Geometry check sheet. Reference: the model listing, model coordinates, mm. A direction names the side the tool comes from. Round coordinates to 2 decimals unless told otherwise and drop trailing zeros. Loops run counter-clockwise (first coordinate to the right, second up) from the corner with the lowest first, then second, coordinate; pieces in that order, holes last.
```python
from build123d import *

# Parameters (mm, degrees)
BOSS_EXTRUDE1_START            = -9
BOSS_EXTRUDE1_DEPTH            = 9
BOSS_EXTRUDE1_2_DEPTH          = 0.4
BOSS_EXTRUDE1_START_2          = -11.95
BOSS_EXTRUDE1_3_DEPTH          = 2.5
SKETCH2_W                      = 9
SKETCH2_H                      = 11
BOSS_EXTRUDE2_DEPTH            = 2.45
SKETCH3_W                      = 0.9
SKETCH3_H                      = 8.5
CUT_EXTRUDE1_DEPTH             = 20.892712233
SKETCH4_W                      = 0.52
SKETCH4_H                      = 6
CUT_EXTRUDE2_DEPTH             = 19.771520983
BOSS_EXTRUDE3_DEPTH            = 0.36
SKETCH6_W                      = 5.62
SKETCH6_H                      = 3
BOSS_EXTRUDE4_DEPTH            = 0.36
SKETCH7_W                      = 3
SKETCH7_H                      = 2.5
BOSS_EXTRUDE5_DEPTH            = 0.52
SKETCH8_W                      = 1.5
SKETCH8_H                      = 1.7
CUT_EXTRUDE3_DEPTH             = 20.7068516
SKETCH9_W                      = 6
SKETCH9_H                      = 1.5
BOSS_EXTRUDE6_DEPTH            = 1.5
SKETCH10_W                     = 10
SKETCH10_H                     = 4.5
CUT_EXTRUDE4_DEPTH             = 20.7068516
BOSS_EXTRUDE7_DEPTH            = 10
BOSS_EXTRUDE8_DEPTH            = 0.25
F_6_5_6_5_DIAMETER_HOLE1_D     = 6.5
F_6_5_6_5_DIAMETER_HOLE1_DEPTH = 7
SKETCH15_W                     = 6
SKETCH15_H                     = 1
SKETCH16_W                     = 0.75
SKETCH16_H                     = 7.825
F_1_5_1_5_DIAMETER_HOLE2_D     = 1.5
F_1_5_1_5_DIAMETER_HOLE3_D     = 1.5
F_1_5_1_5_DIAMETER_HOLE3_DEPTH = 13.88
CHAMFER1_SIZE                  = 0.2


with BuildPart() as part:
    # Boss-Extrude1: read off the stored shape, not the designer's step
    # Boss-Extrude1 outline → Boss-Extrude1 (new body)
    with BuildSketch(Plane(origin=(0, 0, -4.5), x_dir=(-1, 0, 0), z_dir=(0, 0, -1)).offset(BOSS_EXTRUDE1_START)):
        Polygon((11.95, -6.5), (11.95, 4.5), (0, 4.5), (0, -6.5), (9.45, -6.5), align=None)
    extrude(amount=BOSS_EXTRUDE1_DEPTH)

    # Boss-Extrude1 2 outline → Boss-Extrude1 2 (add)
    with BuildSketch(Plane(origin=(0, 0, -4.5), x_dir=(-1, 0, 0), z_dir=(0, 0, -1))):
        with BuildLine():
            Line((11.95, -8.75), (11.95, -6.5))
            Line((11.95, -6.5), (9.45, -6.5))
            Line((9.45, -6.5), (9.45, -8.75))
            ThreePointArc((9.45, -8.75), (10.7, -10), (11.95, -8.75))
        make_face()
    extrude(amount=BOSS_EXTRUDE1_2_DEPTH)

    # Boss-Extrude1 3 outline → Boss-Extrude1 3 (add)
    with BuildSketch(Plane.YZ.offset(BOSS_EXTRUDE1_START_2)):
        with BuildLine():
            Line((-6.5, -4.9), (-3.989897949, -4.9))
            ThreePointArc((-3.989897949, -4.9), (-3.673670183, -4.787298335), (-3.5, -4.5))
            Line((-3.5, -4.5), (-6.5, -4.5))
            Line((-6.5, -4.5), (-6.5, -4.9))
        make_face()
    extrude(amount=BOSS_EXTRUDE1_3_DEPTH)

    # Sketch2 → Boss-Extrude2 (add)
    with BuildSketch(Plane.ZY.offset(11.95)):
        with Locations((0, -1)):
            Rectangle(SKETCH2_W, SKETCH2_H)
    extrude(amount=BOSS_EXTRUDE2_DEPTH)

    # Sketch3 → Cut-Extrude1 (cut, through all)
    with BuildSketch(Plane.XY.offset(4.5)):
        with Locations((-13.95, 0.25)):
            Rectangle(SKETCH3_W, SKETCH3_H)
    extrude(amount=-CUT_EXTRUDE1_DEPTH, mode=Mode.SUBTRACT)

    # Sketch4 → Cut-Extrude2 (cut, through all)
    with BuildSketch(Plane.XZ.offset(6.5)):
        with Locations((-14.14, -1.5)):
            Rectangle(SKETCH4_W, SKETCH4_H)
    extrude(amount=-CUT_EXTRUDE2_DEPTH, mode=Mode.SUBTRACT)

    # Sketch5 → Boss-Extrude3 (add)
    with BuildSketch(Plane(origin=(-13.88, 0, 0), x_dir=(0, -1, 0), z_dir=(-1, 0, 0))):
        with BuildLine():
            Line((6.5, -1.5), (8.5, -1.5))
            ThreePointArc((8.5, -1.5), (10, 0), (8.5, 1.5))
            Line((8.5, 1.5), (6.5, 1.5))
            Line((6.5, 1.5), (6.5, -1.5))
        make_face()
    extrude(amount=-BOSS_EXTRUDE3_DEPTH)

    # Sketch6 → Boss-Extrude4 (add)
    with BuildSketch(Plane(origin=(-13.88, 0, 0), x_dir=(0, -1, 0), z_dir=(-1, 0, 0))):
        with Locations((1.19, 0)):
            Rectangle(SKETCH6_W, SKETCH6_H)
    extrude(amount=-BOSS_EXTRUDE4_DEPTH)

    # Sketch7 → Boss-Extrude5 (add)
    with BuildSketch(Plane.ZY.offset(13.88)):
        with Locations((-3, -5.25)):
            Rectangle(SKETCH7_W, SKETCH7_H)
    extrude(amount=BOSS_EXTRUDE5_DEPTH)

    # Sketch8 → Cut-Extrude3 (cut, through all)
    with BuildSketch(Plane(origin=(0, 0, -4.5), x_dir=(-1, 0, 0), z_dir=(0, 0, -1))):
        with Locations((1.75, 3.65)):
            Rectangle(SKETCH8_W, SKETCH8_H)
    extrude(amount=-CUT_EXTRUDE3_DEPTH, mode=Mode.SUBTRACT)

    # Sketch9 → Boss-Extrude6 (add)
    with BuildSketch(Plane(origin=(-2.5, 0, 0), x_dir=(0, 0, -1), z_dir=(1, 0, 0))):
        with Locations((0, 3.55)):
            Rectangle(SKETCH9_W, SKETCH9_H)
    extrude(amount=BOSS_EXTRUDE6_DEPTH)

    # Sketch10 → Cut-Extrude4 (cut, through all)
    with BuildSketch(Plane(origin=(0, 0, -4.5), x_dir=(-1, 0, 0), z_dir=(0, 0, -1))):
        with Locations((8.5, 2.25)):
            Rectangle(SKETCH10_W, SKETCH10_H)
    extrude(amount=-CUT_EXTRUDE4_DEPTH, mode=Mode.SUBTRACT)

    # Sketch11 → Boss-Extrude7 (add)
    with BuildSketch(Plane.ZY.offset(3.5)):
        with BuildLine():
            Line((4.1, 0), (-4.1, 0))
            ThreePointArc((-4.1, 0), (0, 4.1), (4.1, 0))
        make_face()
    extrude(amount=BOSS_EXTRUDE7_DEPTH)

    # Sketch12 → Boss-Extrude8 (add)
    with BuildSketch(Plane(origin=(-7.825, 0, 0), x_dir=(0, -1, 0), z_dir=(-1, 0, 0))):
        with BuildLine():
            Line((8.75, 1.25), (6.5, 1.25))
            Line((6.5, 1.25), (6.5, -1.25))
            Line((6.5, -1.25), (8.75, -1.25))
            ThreePointArc((8.75, -1.25), (10, 0), (8.75, 1.25))
        make_face()
    extrude(amount=-BOSS_EXTRUDE8_DEPTH)

    # Ø6.5 (6.5) Diameter Hole1
    with Locations(Plane(origin=(0, 0, 0), x_dir=(0, 0, -1), z_dir=(1, 0, 0))):
        with Locations((0, 0)):
            Hole(F_6_5_6_5_DIAMETER_HOLE1_D / 2, depth=F_6_5_6_5_DIAMETER_HOLE1_DEPTH)

    # Sketch15 → Revolve1 (revolve)
    with BuildSketch(Plane.XY, mode=Mode.PRIVATE) as revolve1_sk:
        with Locations((-4, 0.5)):
            Rectangle(SKETCH15_W, SKETCH15_H)
    revolve(revolve1_sk.sketch.rotate(Axis((-7, 0, 0), (1, 0, 0)), 270), axis=Axis((-7, 0, 0), (1, 0, 0)))

    # Sketch16 → Ø1.5 (1.5) Diameter Hole1 (revolve, cut)
    with BuildSketch(Plane(origin=(-7.825, -8.75, 0), x_dir=(0, 0, 1), z_dir=(0, 1, 0))):
        with Locations((0.375, 3.9125)):
            Rectangle(SKETCH16_W, SKETCH16_H)
    revolve(axis=Axis((-14.175, -8.75, 0), (1, 0, 0)), mode=Mode.SUBTRACT)

    # Ø1.5 (1.5) Diameter Hole2 (through all)
    with Locations(Plane.XY.offset(-4.5)):
        with Locations((-10.7, -8.75)):
            Hole(F_1_5_1_5_DIAMETER_HOLE2_D / 2)

    # Ø1.5 (1.5) Diameter Hole3
    with Locations(Plane.ZY.offset(13.88)):
        with Locations((0, -8.75)):
            Hole(F_1_5_1_5_DIAMETER_HOLE3_D / 2, depth=F_1_5_1_5_DIAMETER_HOLE3_DEPTH)

    # Chamfer1
    chamfer1_edges = [part.edges().sort_by_distance(p)[0] for p in [
        (-1, 0, 1),
    ]]
    chamfer(chamfer1_edges, length=CHAMFER1_SIZE)


solid = part.part
```
1) Sectioned sample at C-C, the plane y = -7.5. Record the cut outline in (x, z) (3 decimals).
Report:
outline: (-13.88, -1.5) - (-13.52, -1.5) - (-13.52, 1.5) - (-13.88, 1.5) - close; (-11.95, -4.9) - (-9.45, -4.9) - (-9.45, -4.5) - (-11.95, -4.5) - close; (-7.825, -1.25) - (-7.575, -1.25) - (-7.575, 1.25) - (-7.825, 1.25) - close
2) Gauge pin test, flat ends, axial feed: pin 1 (3 mm diameter, centred on x = -4.5, y = -2, fed in from -Z); pin 2 (3 mm diameter, centred on x = -11, y = -7.5, fed in from +Z); pin 3 (1.4 mm diameter, centred on y = 3.5, z = -1, fed in from -X); pin 4 (4 mm diameter, centred on y = 0, z = 0, fed in from -X). Record the tip position at first contact, or that the pin passes through.
Report:
pin 1: stops at z = -4.5
pin 2: stops at z = 4.5
pin 3: stops at x = -13.5
pin 4: stops at x = -13.88
3) Sectioned sample at A-A, the plane x = -4.5. Record the cut outline in (y, z).
Report:
outline: (-6.5, -4.5) - (0, -4.5) - (0, -4.1) arc R4.1 ccw to (0, 4.1) - (0, 4.5) - (-6.5, 4.5) - close; circle Ø2 at (0, 0); hole circle Ø6.5 at (0, 0)
4) Mould release check, pull along Y, two halves, no side actions. Record for faces 6 (the face through (-13.7, -10, 0)), 7 (the face through (-7, 1, 1)), 8 (the face through (-5, -2, -4.5)): +Y half, -Y half, draft (parallel to the pull), parting line (faces both ways), or undercut.
Report:
face 6: -Y half
face 7: undercut
face 8: draft
5) Sectioned sample at B-B, the plane x = -10.7. Record the cut outline in (y, z), then the cut area to 3 significant figures.
Report:
outline: (-10, -4.9) - (-9.5, -4.9) - (-9.5, -4.5) - (-10, -4.5) - close; (-8, -4.9) - (-3.99, -4.9) arc R0.5 ccw to (-3.5, -4.5) - (0, -4.5) - (0, -4.1) arc R4.1 ccw to (0, 4.1) - (0, 4.5) - (-6.5, 4.5) - (-6.5, -4.5) - (-8, -4.5) - close
area: 86.9 mm2
6) Sectioned sample at D-D, the plane y = -5.25. Record the cut outline in (x, z), then the cut area to 3 significant figures.
Report:
outline: (-14.4, -4.5) - (-11.95, -4.5) - (-11.95, -4.9) - (-9.45, -4.9) - (-9.45, -4.5) - (0, -4.5) - (0, 4.5) - (-14.4, 4.5) - (-14.4, 1.5) - (-13.88, 1.5) - (-13.88, -1.5) - (-14.4, -1.5) - close
area: 129 mm2
7) Access from +Z, -Z, +X, -X, +Y, -Y to the whole of each face (thin tool, end or side, straight path). Record for faces 1 (the face through (-7.575, -7.8, 0)), 2 (the face through (-2, 4, 3)), 3 (the face through (-7.825, -7.8, 0)), 4 (the face through (-2, 4.3, 0)), 5 (the face through (-10.7, -7.8, -4.5)).
Report:
face 1: +Z, -Z, +X, -Y
face 2: +Z, +Y
face 3: +Z, -Z, -Y
face 4: +Z, -Z, +Y
face 5: +Z, +X, -X, -Y
8) Scan lines: line 1 along Y through (x, z) = (-1.5, 0); line 2 along Y through (x, z) = (-13.65, 0); line 3 along Z through (x, y) = (-5, -0.5). Record each from-to range of solid material in increasing order.
Report:
line 1: y = -6.5 to -3.25, -1 to 1, 3.25 to 4.3
line 2: y = -10 to -9.5, -8 to 1.62
line 3: z = -4.5 to -3.21, -0.87 to 0.87, 3.21 to 4.5
